```python
from build123d import *

# Parameters (mm, degrees)
F1_DEPTH      = 25
F1_DEPTH_BACK = 25
F2_DEPTH      = 25
F4_D          = 5


with BuildPart() as f1:
    # F0 (on Right) → F1 (new body, two sides)
    with BuildSketch(Plane.YZ) as f1_sk:
        Polygon((48.1754057109, 59.2439547181), (-58.3366975188, 41.8245978653), (-12.4294357374, 6.8044359796), (58.1552386284, 19.687499851), align=None)
    extrude(amount=F1_DEPTH)
    extrude(f1_sk.sketch, amount=-F1_DEPTH_BACK)

    # F2 (add): a face of the model
    f2_faces = [f1.faces().sort_by_distance(p)[0] for p in [
        (0, 22.8629014455, 13.2459679153),
    ]]
    extrude(f2_faces, amount=F2_DEPTH)

    # F4 (through all)
    with Locations(Plane(origin=(-25, 0, 0), x_dir=(0, -1, 0), z_dir=(-1, 0, 0))):
        with Locations((-23.3555603772, 20.5315314233)):
            Hole(F4_D / 2)


solid = f1.part
```
The listing builds one solid part. Answer for the finished solid, in the listing's coordinates (mm). Give positions to 0.01 mm unless a question says otherwise; leave off trailing zeros. Order: outer loops, then holes, each group sorted by start corner. A loop starts at its lowest first (then second) coordinate and runs counter-clockwise, first axis right, second up. Notation, with made-up numbers: (29.25, -38) -> (68.25, -38) arc R23 ccw to (68.25, -13) -> close; hole circle Ø10 at (55.25, 3). An arc over 180 degrees is marked (long way). Answer as a JSON object with one key per item and string values. Group by question number.
Item 1: Consider L1, parallel to Z at x = 19, y = 22; L2, parallel to Z at x = 2.5, y = 7; L3, parallel to Z at x = 16.5, y = -49.5. Determine where each line is inside the solid, lowest interval first. Write a range as from..to.
Item 2: The part is cut by section A-A on x = -2. Write down the section's boundary in (y, z), and give its area (3 significant figures).
Item 3: The part is cut by section C-C on z = 11. Write down the section's boundary in (x, y), and give its area (3 significant figures).
Item 4: Flat-ended cylindrical pins translate along their axes: pin 1 (4 mm diameter, centred on x = 12, y = -1, fed in from +Z); pin 2 (5 mm diameter, centred on x = 5.5, y = 43.5, fed in from +Z); pin 3 (2 mm diameter, centred on x = 15, y = -39, fed in from +Z). Find the tip coordinate at first contact, or state that the pin passes through.
Item 5: The part is cut by section B-B on y = -15. Write down the section's boundary in (x, z).
Item 6: Determine the mould class of faces 1 (the flat face through (-25, 13, 21)), 2 (the flat face through (0.35, -35.704, 24.56)), 3 (the flat face through (0.35, 60.37, 7.56)), 4 (the cylindrical face through (0.35, 21.37, 19.01)) for opening direction Y: pulls with the +Y half, pulls with the -Y half, needs draft (parallel to the pull), parting line crosses it, or undercut.
Result set:
{
 "1": {"L1": "-12.32..18.43, 22.63..54.96", "L2": "-15.06..52.51", "L3": "35.08..43.27"},
 "2": {"outline": "(-58.34, 41.82) -> (-12.43, 6.8) -> (-7.94, -17.79) -> (62.64, -4.91) -> (58.16, 19.69) -> (48.18, 59.24) -> close; hole circle Ø5 at (23.36, 20.53)", "area": "5,500 mm²"},
 "3": {"outline": "(-25, -17.93) -> (25, -17.93) -> (25, 59.74) -> (-25, 59.74) -> close", "area": "3,880 mm²"},
 "4": {"pin 1": "z = 51.53", "pin 2": "z = 58.89", "pin 3": "z = 45.15"},
 "5": {"outline": "(-25, 8.77) -> (25, 8.77) -> (25, 48.91) -> (-25, 48.91) -> close"},
 "6": {"face 1": "needs draft", "face 2": "pulls with the -Y half", "face 3": "pulls with the +Y half", "face 4": "undercut"}
}
